The listing builds one solid part. Answer for the finished solid, in the listing's coordinates (mm). Round coordinates to 2 decimals unless told otherwise and drop trailing zeros. Write each loop counter-clockwise with the first axis right and the second up, starting at its lowest first coordinate (ties: lowest second). Pieces come first, ordered by that corner, then holes. Notation, with made-up numbers: (-30, -12) - (7, -12) arc R24 cw to (7, -1) - close; hole circle Ø8 at (-16, -18). An arc over 180 degrees is marked (long way). Return JSON: item names as keys, results as strings. Group by question number.
(1) Section B-B, the plane x = 49 is taken. Write down the section's boundary in (y, z).
(2) Each of these flat-tipped pins is pushed along its axis until it touches: pin 1 (4 mm diameter, centred on x = 39.5, z = 17.5, fed in from +Y); pin 2 (2 mm diameter, centred on y = 16.5, z = 0, fed in from +X); pin 3 (20.5 mm diameter, centred on x = 21, y = -7, fed in from +Z). Where does it stop, or does it pass through?
(3) Determine the mould class of faces 1 (the flat face through (-8, 0, 0)), 2 (the cylindrical face through (65.49, 0.28, -87.37)), 3 (the cylindrical face through (-78.94, 23.87, -43.91)) for opening direction Z: +Z half, -Z half, draft (parallel to the pull), parting line (faces both ways), or undercut.
(4) Section C-C, the plane y = -18 is taken. Write down the section's boundary in (x, z).
(5) Find the intervals of material crossed by line 1 along Z through (x, y) = (-73, 19.5); line 2 along X through (y, z) = (1, 10.5); line 3 along X through (y, z) = (6, 15.5), in increasing order. Write a range as [from, to].
(6) Section A-A, the plane y = 4 is taken. Write down the section's boundary in (x, z), then the cut area to 3 significant figures.
```python
from build123d import *

# Parameters (mm, degrees)
F1_R         = 9.6860400986
F3_W         = 147.32
F3_H         = 88.9
F4_DEPTH     = 25.4
F5_R         = 5.08
F6_T1_DEPTH  = 40.64
F6_S5_W      = 5.08
F6_S5_H      = 5.08
F6_T6_DEPTH  = 5.08
F6_S11_W     = 5.08
F6_S11_H     = 5.08
F6_T12_DEPTH = 5.08
F7_T1_DEPTH  = 40.64
F7_S5_W      = 5.08
F7_S5_H      = 5.08
F7_T6_DEPTH  = 5.08
F7_S11_W     = 5.08
F7_S11_H     = 5.08
F7_T12_DEPTH = 5.08
F8_T1_DEPTH  = 40.64
F8_T3_DEPTH  = 137.16
F8_S7_W      = 5.08
F8_S7_H      = 5.08
F8_T8_DEPTH  = 5.08
F8_S13_W     = 5.08
F8_S13_H     = 5.08
F8_T14_DEPTH = 5.08
F8_T18_ANGLE = 90
F8_T20_ANGLE = 90


# Not quite as in the source:
# - a fillet or chamfer that OpenCascade refuses, or shapes differently, is made with other operations: its cross-section is extruded or revolved along the edge and cut away or added


with BuildPart() as f2:
    # F2: sweep along a path in F0
    with BuildLine(Plane.XZ) as f2_path:
        ThreePointArc((37.5847704709, 0), (-4.2709950358, 41.8557655066), (-46.1267605424, 0))
    # F1 (on Top) → F2 (sweep)
    with BuildSketch(Plane.XY):
        with Locations((37.5847704709, 0)):
            Circle(F1_R)
    sweep(path=f2_path.line)

    # F3 (on Front) → F4 (join, symmetric)
    with BuildSketch(Plane.XZ):
        with Locations((-6.7246720757, -44.45)):
            Rectangle(F3_W, F3_H)
    extrude(amount=F4_DEPTH, both=True)

    # F5
    f5_edges = [f2.edges().sort_by_distance(p)[0] for p in [
        (-80.384672, -25.4, -44.45),
        (66.935328, -25.4, -44.45),
        (66.935328, 25.4, -44.45),
        (-80.384672, 25.4, -44.45),
        (-6.724672, 25.4, 0),
        (-6.724672, -25.4, -88.9),
        (-6.724672, -25.4, 0),
    ]]
    fillet(f5_edges, radius=F5_R)

    # F6: fillet of radius 5.08 on 1 edges, made by hand

    # F6_s2 → F6_t1 (cut)
    with BuildSketch(Plane.XZ.offset(-20.32)):
        with BuildLine():
            ThreePointArc((61.8553279243, 0), (65.4474303727, -1.4878975516), (66.9353279243, -5.08))
            Line((66.9353279243, -5.08), (66.9353279243, 0))
            Line((66.9353279243, 0), (61.8553279243, 0))
        make_face()
    extrude(amount=F6_T1_DEPTH, mode=Mode.SUBTRACT)


with BuildPart() as f6_tool4:
    # F6_s5 → F6_t6 (new body)
    with BuildSketch(Plane.XY.offset(-5.08)):
        with Locations((64.3953279243, -22.86)):
            Rectangle(F6_S5_W, F6_S5_H)
    extrude(amount=F6_T6_DEPTH)

    # F6_s7 → F6_t8 (revolve, cut)
    with BuildSketch(Plane(origin=(61.8553279243, -20.32, -5.08), x_dir=(-0.7071067812, 0.7071067812, 0), z_dir=(0.7071067812, 0.7071067812, 0))):
        with BuildLine():
            ThreePointArc((0, -5.08), (5.08, 0), (0, 5.08))
            Line((0, 5.08), (0, -5.08))
        make_face()
    revolve(axis=Axis((61.8553279243, -20.32, -5.08), (0, 0, 1)), mode=Mode.SUBTRACT)


with BuildPart() as f2_1:
    add(f2.part)

    # F6_t3: cut F6_tool4
    add(f6_tool4.part, mode=Mode.SUBTRACT)


with BuildPart() as f6_tool10:
    # F6_s11 → F6_t12 (new body)
    with BuildSketch(Plane.XY.offset(-5.08)):
        with Locations((64.3953279243, 22.86)):
            Rectangle(F6_S11_W, F6_S11_H)
    extrude(amount=F6_T12_DEPTH)

    # F6_s13 → F6_t14 (revolve, cut)
    with BuildSketch(Plane(origin=(61.8553279243, 20.32, -5.08), x_dir=(-0.7071067812, -0.7071067812, 0), z_dir=(-0.7071067812, 0.7071067812, 0))):
        with BuildLine():
            ThreePointArc((0, -5.08), (5.08, 0), (0, 5.08))
            Line((0, 5.08), (0, -5.08))
        make_face()
    revolve(axis=Axis((61.8553279243, 20.32, -5.08), (0, 0, 1)), mode=Mode.SUBTRACT)


with BuildPart() as f2_2:
    add(f2_1.part)

    # F6_t9: cut F6_tool10
    add(f6_tool10.part, mode=Mode.SUBTRACT)

    # F7: fillet of radius 5.08 on 1 edges, made by hand

    # F7_s2 → F7_t1 (cut)
    with BuildSketch(Plane.XZ.offset(-20.32)):
        with BuildLine():
            ThreePointArc((-75.3046720757, 0), (-78.8967745241, -1.4878975516), (-80.3846720757, -5.08))
            Line((-80.3846720757, -5.08), (-80.3846720757, 0))
            Line((-80.3846720757, 0), (-75.3046720757, 0))
        make_face()
    extrude(amount=F7_T1_DEPTH, mode=Mode.SUBTRACT)


with BuildPart() as f7_tool4:
    # F7_s5 → F7_t6 (new body)
    with BuildSketch(Plane.XY.offset(-5.08)):
        with Locations((-77.8446720757, 22.86)):
            Rectangle(F7_S5_W, F7_S5_H)
    extrude(amount=F7_T6_DEPTH)

    # F7_s7 → F7_t8 (revolve, cut)
    with BuildSketch(Plane(origin=(-75.3046720757, 20.32, -5.08), x_dir=(0.7071067812, -0.7071067812, 0), z_dir=(-0.7071067812, -0.7071067812, 0))):
        with BuildLine():
            ThreePointArc((0, -5.08), (5.08, 0), (0, 5.08))
            Line((0, 5.08), (0, -5.08))
        make_face()
    revolve(axis=Axis((-75.3046720757, 20.32, -5.08), (0, 0, 1)), mode=Mode.SUBTRACT)


with BuildPart() as f2_3:
    add(f2_2.part)

    # F7_t3: cut F7_tool4
    add(f7_tool4.part, mode=Mode.SUBTRACT)


with BuildPart() as f7_tool10:
    # F7_s11 → F7_t12 (new body)
    with BuildSketch(Plane.XY.offset(-5.08)):
        with Locations((-77.8446720757, -22.86)):
            Rectangle(F7_S11_W, F7_S11_H)
    extrude(amount=F7_T12_DEPTH)

    # F7_s13 → F7_t14 (revolve, cut)
    with BuildSketch(Plane(origin=(-75.3046720757, -20.32, -5.08), x_dir=(0.7071067812, 0.7071067812, 0), z_dir=(0.7071067812, -0.7071067812, 0))):
        with BuildLine():
            ThreePointArc((0, -5.08), (5.08, 0), (0, 5.08))
            Line((0, 5.08), (0, -5.08))
        make_face()
    revolve(axis=Axis((-75.3046720757, -20.32, -5.08), (0, 0, 1)), mode=Mode.SUBTRACT)


with BuildPart() as f2_4:
    add(f2_3.part)

    # F7_t9: cut F7_tool10
    add(f7_tool10.part, mode=Mode.SUBTRACT)

    # F8: fillet of radius 5.08 on 1 edges, made by hand

    # F8_s2 → F8_t1 (cut)
    with BuildSketch(Plane.XZ.offset(-20.32)):
        with BuildLine():
            ThreePointArc((-80.3846720757, -83.82), (-78.8967745241, -87.4121024484), (-75.3046720757, -88.9))
            Line((-75.3046720757, -88.9), (-80.3846720757, -88.9))
            Line((-80.3846720757, -88.9), (-80.3846720757, -83.82))
        make_face()
        with BuildLine():
            ThreePointArc((66.9353279243, -83.82), (65.4474303727, -87.4121024484), (61.8553279243, -88.9))
            Line((61.8553279243, -88.9), (66.9353279243, -88.9))
            Line((66.9353279243, -88.9), (66.9353279243, -83.82))
        make_face()
    extrude(amount=F8_T1_DEPTH, mode=Mode.SUBTRACT)

    # F8_s4 → F8_t3 (cut)
    with BuildSketch(Plane.YZ.offset(-75.3046720757)):
        with BuildLine():
            ThreePointArc((25.4, -83.82), (23.9121024484, -87.4121024484), (20.32, -88.9))
            Line((20.32, -88.9), (25.4, -88.9))
            Line((25.4, -88.9), (25.4, -83.82))
        make_face()
    extrude(amount=F8_T3_DEPTH, mode=Mode.SUBTRACT)


with BuildPart() as f8_tool6:
    # F8_s7 → F8_t8 (new body)
    with BuildSketch(Plane.YZ.offset(-75.3046720757)):
        with Locations((-22.86, -86.36)):
            Rectangle(F8_S7_W, F8_S7_H)
    extrude(amount=-F8_T8_DEPTH)

    # F8_s9 → F8_t10 (revolve, cut)
    with BuildSketch(Plane(origin=(-75.3046720757, -20.32, -83.82), x_dir=(0, 0.7071067812, 0.7071067812), z_dir=(0, -0.7071067812, 0.7071067812))):
        with BuildLine():
            ThreePointArc((0, -5.08), (5.08, 0), (0, 5.08))
            Line((0, 5.08), (0, -5.08))
        make_face()
    revolve(axis=Axis((-75.3046720757, -20.32, -83.82), (-1, 0, 0)), mode=Mode.SUBTRACT)


with BuildPart() as f2_5:
    add(f2_4.part)

    # F8_t5: cut F8_tool6
    add(f8_tool6.part, mode=Mode.SUBTRACT)


with BuildPart() as f8_tool12:
    # F8_s13 → F8_t14 (new body)
    with BuildSketch(Plane.YZ.offset(61.8553279243)):
        with Locations((-22.86, -86.36)):
            Rectangle(F8_S13_W, F8_S13_H)
    extrude(amount=F8_T14_DEPTH)

    # F8_s15 → F8_t16 (revolve, cut)
    with BuildSketch(Plane(origin=(61.8553279243, -20.32, -83.82), x_dir=(0, 0.7071067812, 0.7071067812), z_dir=(0, 0.7071067812, -0.7071067812))):
        with BuildLine():
            ThreePointArc((0, -5.08), (5.08, 0), (0, 5.08))
            Line((0, 5.08), (0, -5.08))
        make_face()
    revolve(axis=Axis((61.8553279243, -20.32, -83.82), (1, 0, 0)), mode=Mode.SUBTRACT)


with BuildPart() as f2_6:
    add(f2_5.part)

    # F8_t11: cut F8_tool12
    add(f8_tool12.part, mode=Mode.SUBTRACT)

    # F8_s17 → F8_t18 (revolve, cut)
    with BuildSketch(Plane.YZ.offset(-75.3046720757)):
        with BuildLine():
            ThreePointArc((20.32, -88.9), (23.9121024484, -87.4121024484), (25.4, -83.82))
            Line((25.4, -83.82), (25.4, -88.9))
            Line((25.4, -88.9), (20.32, -88.9))
        make_face()
    revolve(axis=Axis((-75.3046720757, 20.32, -88.9), (0, 0, 1)), revolution_arc=F8_T18_ANGLE, mode=Mode.SUBTRACT)

    # F8_s19 → F8_t20 (revolve, cut)
    with BuildSketch(Plane.YZ.offset(61.8553279243)):
        with BuildLine():
            ThreePointArc((20.32, -88.9), (23.9121024484, -87.4121024484), (25.4, -83.82))
            Line((25.4, -83.82), (25.4, -88.9))
            Line((25.4, -88.9), (20.32, -88.9))
        make_face()
    revolve(axis=Axis((61.8553279243, 20.32, -88.9), (0, 0, -1)), revolution_arc=F8_T20_ANGLE, mode=Mode.SUBTRACT)


solid = f2_6.part
```
Working result:
{
 "1": {"outline": "(-25.4, -83.82) arc R5.08 ccw to (-20.32, -88.9) - (20.32, -88.9) arc R5.08 ccw to (25.4, -83.82) - (25.4, -5.08) arc R5.08 ccw to (20.32, 0) - (-20.32, 0) arc R5.08 ccw to (-25.4, -5.08) - close"},
 "2": {"pin 1": "stops at y = 9.11", "pin 2": "stops at x = 64.88", "pin 3": "stops at z = 48.67"},
 "3": {"face 1": "undercut", "face 2": "-Z half", "face 3": "draft"},
 "4": {"outline": "(-80.38, -83.82) arc R5.08 ccw to (-75.3, -88.9) - (61.86, -88.9) arc R5.08 ccw to (66.94, -83.82) - (66.94, -5.08) arc R5.08 ccw to (61.86, 0) - (-75.3, 0) arc R5.08 ccw to (-80.38, -5.08) - close"},
 "5": {"line 1": "z = [-88.9, 0]", "line 2": "x = [-54.68, -34.73], [26.19, 46.14]", "line 3": "x = [-51.24, -34.82], [26.27, 42.7]"},
 "6": {"outline": "(-80.38, -83.82) arc R5.08 ccw to (-75.3, -88.9) - (61.86, -88.9) arc R5.08 ccw to (66.94, -83.82) - (66.94, -5.08) arc R5.08 ccw to (61.86, 0) - (46.41, 0) arc R50.68 ccw to (-54.95, 0) - (-75.3, 0) arc R5.08 ccw to (-80.38, -5.08) - close; hole (-37.31, 0) - (28.76, 0) arc R33.03 ccw to start", "area": "15,400 mm^2"}
}
